Geometry: final body of the model. Coordinates: model frame, mm. A direction names the side the tool comes from. Coordinates: 2 decimals unless noted, no trailing zeros. Write each loop counter-clockwise with the first axis right and the second up, starting at its lowest first coordinate (ties: lowest second). Pieces come first, ordered by that corner, then holes. Notation, with made-up numbers: (-35, -29) - (20, -29) arc R30 cw to (20, 3) - close; hole circle Ø4 at (-3.5, 20). An arc over 180 degrees is marked (long way). Answer as a JSON object with one key per item and string values. Group by question number.
Item 1: Section A-A on x = -36.5. Return loops of the section in (y, z), and give its area (4 significant figures).
Item 2: Line query: line 1 along X through (y, z) = (2.2, -29); line 2 along Z through (x, y) = (-2.5, 0.25); line 3 along Z through (x, y) = (27, 0.6). Output: solid intervals per line, ascending. Write a range as from..to.
Item 3: Section B-B on x = 23. Return loops of the section in (y, z), and give its area (3 significant figures).
Item 4: Section C-C on x = -18. Return loops of the section in (y, z).
Item 5: Mould query, pull axis Z, two halves, no side actions, for faces 4 (the flat face through (1, 1, -32.5)), 5 (the flat face through (-40, 1, 28)), 6 (the flat face through (11, 1, 21.8)), 7 (the flat face through (1.75, 1, -29)). Classes: pulls with the +Z half, pulls with the -Z half, needs draft (parallel to the pull), parting line crosses it, or undercut.
Item 6: Set-up query: faces 1 (the flat face through (-30, 1, 23.5)), 2 (the flat face through (40, 1, 0)), 3 (the flat face through (0, 1, -27.5)). Return all of +Z, -Z, +X, -X, +Y, -Y with unobstructed straight access to the full face (end or side cutting, diameter ignored); none if empty.
Item 7: Section D-D on z = -29. Return loops of the section in (x, y), and give its area (4 significant figures).
```python
from build123d import *

# Parameters (mm, degrees)
CROQUIS1_R              = 1
CROQUIS1_W              = 3
CROQUIS1_H              = 3.5
CROQUIS1_W_2            = 3.5
CROQUIS1_H_2            = 3
SALIENTE_EXTRUIR1_DEPTH = 3


with BuildPart() as part:
    # Croquis1 → Saliente-Extruir1 (new body)
    with BuildSketch(Plane(origin=(0, 0, 0), x_dir=(1, 0, 0), z_dir=(0, 1, 0))):
        with BuildLine():
            Line((-39, -32.5), (39, -32.5))
            ThreePointArc((39, -32.5), (39.707106781, -32.207106781), (40, -31.5))
            Line((40, -31.5), (40, 31.5))
            ThreePointArc((40, 31.5), (39.707106781, 32.207106781), (39, 32.5))
            Line((39, 32.5), (-39, 32.5))
            ThreePointArc((-39, 32.5), (-39.707106781, 32.207106781), (-40, 31.5))
            Line((-40, 31.5), (-40, -12.5))
            ThreePointArc((-40, -12.5), (-39.707106781, -13.207106781), (-39, -13.5))
            Line((-39, -13.5), (-21, -13.5))
            ThreePointArc((-21, -13.5), (-20.292893219, -13.792893219), (-20, -14.5))
            Line((-20, -14.5), (-20, -22.5))
            ThreePointArc((-20, -22.5), (-20.292893219, -23.207106781), (-21, -23.5))
            Line((-21, -23.5), (-39, -23.5))
            ThreePointArc((-39, -23.5), (-39.707106781, -23.792893219), (-40, -24.5))
            Line((-40, -24.5), (-40, -31.5))
            ThreePointArc((-40, -31.5), (-39.707106781, -32.207106781), (-39, -32.5))
        make_face()
        with Locations(Location((-36.5, 29, 0), (0, 0, 270))):
            Circle(CROQUIS1_R, mode=Mode.SUBTRACT)
        with Locations(Location((-36.5, -29, 0), (0, 0, 270))):
            Circle(CROQUIS1_R, mode=Mode.SUBTRACT)
        with Locations(Location((36.5, 29, 0), (0, 0, 270))):
            Circle(CROQUIS1_R, mode=Mode.SUBTRACT)
        with Locations(Location((36.5, -29, 0), (0, 0, 270))):
            Circle(CROQUIS1_R, mode=Mode.SUBTRACT)
        with Locations((-36.5, 0)):
            Rectangle(CROQUIS1_W, CROQUIS1_H, mode=Mode.SUBTRACT)
        with Locations((36.5, 0)):
            Rectangle(CROQUIS1_W, CROQUIS1_H, mode=Mode.SUBTRACT)
        with Locations((0, -29)):
            Rectangle(CROQUIS1_W_2, CROQUIS1_H_2, mode=Mode.SUBTRACT)
        with Locations((0, 29)):
            Rectangle(CROQUIS1_W_2, CROQUIS1_H_2, mode=Mode.SUBTRACT)
        with BuildLine():
            Line((-10, -26.8), (32, -26.8))
            ThreePointArc((32, -26.8), (32.707106781, -26.507106781), (33, -25.8))
            Line((33, -25.8), (33, -22.8))
            ThreePointArc((33, -22.8), (32.707106781, -22.092893219), (32, -21.8))
            Line((32, -21.8), (-10, -21.8))
            ThreePointArc((-10, -21.8), (-10.707106781, -22.092893219), (-11, -22.8))
            Line((-11, -22.8), (-11, -25.8))
            ThreePointArc((-11, -25.8), (-10.707106781, -26.507106781), (-10, -26.8))
        make_face(mode=Mode.SUBTRACT)
        with BuildLine():
            Line((26, 6.5), (31, 6.5))
            ThreePointArc((31, 6.5), (31.707106781, 6.207106781), (32, 5.5))
            Line((32, 5.5), (32, -2.5))
            ThreePointArc((32, -2.5), (31.707106781, -3.207106781), (31, -3.5))
            Line((31, -3.5), (26, -3.5))
            ThreePointArc((26, -3.5), (25.292893219, -3.207106781), (25, -2.5))
            Line((25, -2.5), (25, 5.5))
            ThreePointArc((25, 5.5), (25.292893219, 6.207106781), (26, 6.5))
        make_face(mode=Mode.SUBTRACT)
        with BuildLine():
            Line((-21, 26.8), (32, 26.8))
            ThreePointArc((32, 26.8), (32.707106781, 26.507106781), (33, 25.8))
            Line((33, 25.8), (33, 22.8))
            ThreePointArc((33, 22.8), (32.707106781, 22.092893219), (32, 21.8))
            Line((32, 21.8), (-21, 21.8))
            ThreePointArc((-21, 21.8), (-21.707106781, 22.092893219), (-22, 22.8))
            Line((-22, 22.8), (-22, 25.8))
            ThreePointArc((-22, 25.8), (-21.707106781, 26.507106781), (-21, 26.8))
        make_face(mode=Mode.SUBTRACT)
        with BuildLine():
            Line((-32, 26.8), (-24, 26.8))
            ThreePointArc((-24, 26.8), (-23.292893219, 26.507106781), (-23, 25.8))
            Line((-23, 25.8), (-23, 17.8))
            ThreePointArc((-23, 17.8), (-23.292893219, 17.092893219), (-24, 16.8))
            Line((-24, 16.8), (-32, 16.8))
            ThreePointArc((-32, 16.8), (-32.707106781, 17.092893219), (-33, 17.8))
            Line((-33, 17.8), (-33, 25.8))
            ThreePointArc((-33, 25.8), (-32.707106781, 26.507106781), (-32, 26.8))
        make_face(mode=Mode.SUBTRACT)
    extrude(amount=SALIENTE_EXTRUIR1_DEPTH)


solid = part.part
```
Checks:
{
 "1": {"outline": "(0, -32.5) - (3, -32.5) - (3, -30) - (0, -30) - close; (0, -28) - (3, -28) - (3, -1.75) - (0, -1.75) - close; (0, 1.75) - (3, 1.75) - (3, 13.5) - (0, 13.5) - close; (0, 23.5) - (3, 23.5) - (3, 28) - (0, 28) - close; (0, 30) - (3, 30) - (3, 32.5) - (0, 32.5) - close", "area": "142.5 mm^2"},
 "2": {"line 1": "-40..-37.5, -35.5..-1.75, 1.75..35.5, 37.5..40", "line 2": "-32.5..-26.8, -21.8..21.8, 26.8..32.5", "line 3": "-32.5..-26.8, -21.8..-6.5, 3.5..21.8, 26.8..32.5"},
 "3": {"outline": "(0, -32.5) - (3, -32.5) - (3, -26.8) - (0, -26.8) - close; (0, -21.8) - (3, -21.8) - (3, 21.8) - (0, 21.8) - close; (0, 26.8) - (3, 26.8) - (3, 32.5) - (0, 32.5) - close", "area": "165 mm^2"},
 "4": {"outline": "(0, -32.5) - (3, -32.5) - (3, -26.8) - (0, -26.8) - close; (0, -21.8) - (3, -21.8) - (3, 32.5) - (0, 32.5) - close"},
 "5": {"face 4": "pulls with the -Z half", "face 5": "needs draft", "face 6": "undercut", "face 7": "undercut"},
 "6": {"face 1": "-X, +Y, -Y", "face 2": "+Z, -Z, +X, +Y, -Y", "face 3": "+Y, -Y"},
 "7": {"outline": "(-40, 0) - (-37.5, 0) - (-37.5, 3) - (-40, 3) - close; (-35.5, 0) - (-1.75, 0) - (-1.75, 3) - (-35.5, 3) - close; (1.75, 0) - (35.5, 0) - (35.5, 3) - (1.75, 3) - close; (37.5, 0) - (40, 0) - (40, 3) - (37.5, 3) - close", "area": "217.5 mm^2"}
}
